Design review of the part built by this model. Coordinates are the model's own, in mm. Face numbers are marked on the shaded views. Coordinates: 2 decimals unless noted, no trailing zeros. Loops run counter-clockwise (first coordinate to the right, second up) from the corner with the lowest first, then second, coordinate; pieces in that order, holes last. Notation, with made-up numbers: (-31, 29) -> (-24, 29) arc R20 cw to (-24, 39) -> close; hole circle Ø6 at (78.5, 46.5). An arc over 180 degrees is marked (long way). Answer in a Markdown table with one row per item.
```python
from build123d import *

# Parameters (mm, degrees)
F0_W     = 100
F0_H     = 80
F1_DEPTH = 15
F2_W     = 86
F2_H     = 66
F3_DEPTH = 11
F4_W     = 79
F4_H     = 59
F5_DEPTH = 4.001


with BuildPart() as f1:
    # F0 (on Top) → F1 (new body)
    with BuildSketch(Plane.XY):
        Rectangle(F0_W, F0_H)
    extrude(amount=F1_DEPTH)

    # F2 (on face) → F3 (cut)
    with BuildSketch(Plane.XY.offset(15)):
        Rectangle(F2_W, F2_H)
    extrude(amount=-F3_DEPTH, mode=Mode.SUBTRACT)

    # F4 (on face) → F5 (cut, through all)
    with BuildSketch(Plane.XY.offset(4)):
        Rectangle(F4_W, F4_H)
    extrude(amount=-F5_DEPTH, mode=Mode.SUBTRACT)


solid = f1.part
```
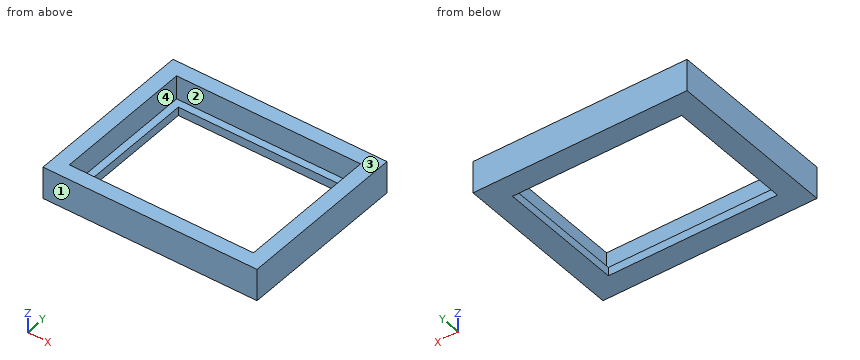
(1) To check wall thickness, follow probe 1 along X at (y, z) = (-2, 4.5); probe 2 along Y at (x, z) = (-8.5, 9.25); probe 3 along Y at (x, z) = (13, 3). State the ranges of each line that lie inside material, in increasing order.
Evaluation:
| item | result |
|---|---|
| probe 1 | x = -50 to -43, 43 to 50 |
| probe 2 | y = -40 to -33, 33 to 40 |
| probe 3 | y = -40 to -29.5, 29.5 to 40 |
(2) Take a section at D-D on x = 41.5. Give the boundary of the cut face in (y, z), and give its area (3 significant figures).
Evaluation:
| item | result |
|---|---|
| outline | (-40, 0) -> (40, 0) -> (40, 15) -> (33, 15) -> (33, 4) -> (-33, 4) -> (-33, 15) -> (-40, 15) -> close |
| area | 474 mm² |
(3) Take a section at C-C on z = 13.5. Give the boundary of the cut face in (x, y).
Evaluation:
| item | result |
|---|---|
| outline | (-50, -40) -> (50, -40) -> (50, 40) -> (-50, 40) -> close; hole (-43, -33) -> (43, -33) -> (43, 33) -> (-43, 33) -> close |
(4) Take a section at A-A on y = 14. Give the boundary of the cut face in (x, z).
Evaluation:
| item | result |
|---|---|
| outline | (-50, 0) -> (-39.5, 0) -> (-39.5, 4) -> (-43, 4) -> (-43, 15) -> (-50, 15) -> close; (39.5, 0) -> (50, 0) -> (50, 15) -> (43, 15) -> (43, 4) -> (39.5, 4) -> close |
(5) Draft analysis for pull direction Y (two halves, no side actions). For the marked faces 1, 2, 3 and 4, state which applies: pulls with the +Y half, pulls with the -Y half, needs draft (parallel to the pull), parting line crosses it, or undercut.
Evaluation:
| item | result |
|---|---|
| face 1 | pulls with the -Y half |
| face 2 | undercut |
| face 3 | needs draft |
| face 4 | undercut |
(6) Take a section at B-B on x = 7.5. Give the boundary of the cut face in (y, z), and give its area (3 significant figures).
Evaluation:
| item | result |
|---|---|
| outline | (-40, 0) -> (-29.5, 0) -> (-29.5, 4) -> (-33, 4) -> (-33, 15) -> (-40, 15) -> close; (29.5, 0) -> (40, 0) -> (40, 15) -> (33, 15) -> (33, 4) -> (29.5, 4) -> close |
| area | 238 mm² |
